Build history of the part. All positions in model axes, mm. Round coordinates to 2 decimals unless told otherwise and drop trailing zeros. Use a Markdown table: item, result.
from build123d import *

# Parameters (mm, degrees)
SKETCH1_W           = 492
SKETCH1_H           = 45
BOSS_EXTRUDE1_DEPTH = 3
SKETCH2_W           = 3
SKETCH2_H           = 30
CUT_EXTRUDE1_DEPTH  = 4
LPATTERN1_COUNT     = 14
LPATTERN1_PITCH     = 33


with BuildPart() as part:
    # Sketch1 → Boss-Extrude1 (new body)
    with BuildSketch(Plane.XY):
        Rectangle(SKETCH1_W, SKETCH1_H)
    extrude(amount=BOSS_EXTRUDE1_DEPTH)

    # Sketch2 → Cut-Extrude1 (cut, through all)
    with BuildSketch(Plane.XY.offset(3)):
        with Locations((-214.5, -7.5)):
            Rectangle(SKETCH2_W, SKETCH2_H)
    cut_extrude1 = extrude(amount=-CUT_EXTRUDE1_DEPTH, mode=Mode.SUBTRACT)

    # LPattern1: Cut-Extrude1 ×14
    with Locations(*[(i * LPATTERN1_PITCH, 0, 0) for i in range(1, LPATTERN1_COUNT)]):
        add(cut_extrude1, mode=Mode.SUBTRACT)


solid = part.part
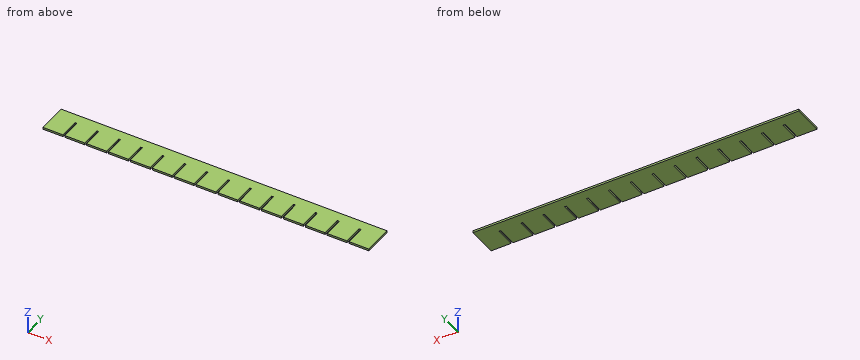
Q1. Probe line 1 (Y direction, x = -215.5, z = 1.85). List the from-to ranges inside material, lowest first.
Results found:
| item | result |
|---|---|
| line 1 | y = 7.5 to 22.5 |
Q2. Drop a flat-ended pin along its axis: pin 1 (1.5 mm diameter, centred on x = -181.5, z = 2, fed in from -Y). Give the stop position or say it passes through.
Results found:
| item | result |
|---|---|
| pin 1 | stops at y = 7.5 |
Q3. Cut at A-A, the plane y = 1. Count the separate pieces of the cut face and the enclosed holes in it, plus the area to 3 significant figures.
Results found:
| item | result |
|---|---|
| separate pieces | 15 |
| enclosed holes | 0 |
| area | 1,350 mm2 |
